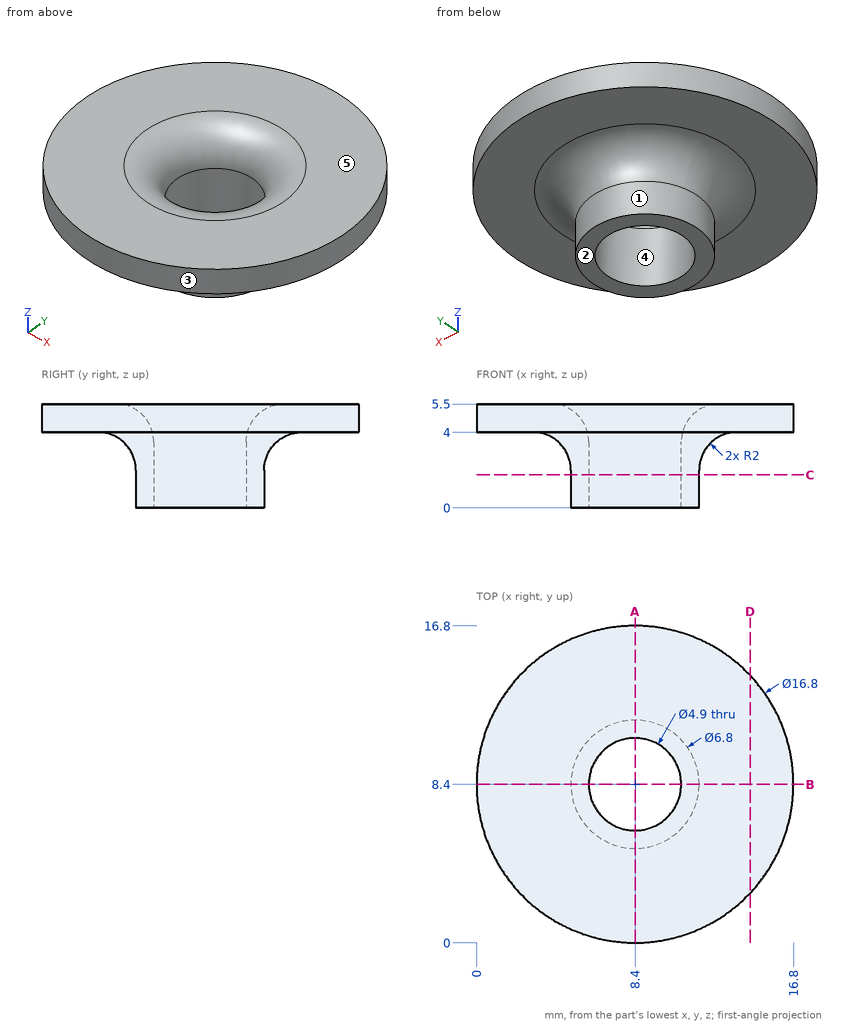
Geometry: see drawing. Coordinates: mm, zero at the bounding-box minimum. A direction names the side the tool comes from. Round coordinates to 2 decimals unless told otherwise and drop trailing zeros. Loops run counter-clockwise (first coordinate to the right, second up) from the corner with the lowest first, then second, coordinate; pieces in that order, holes last. Notation, with made-up numbers: M 28,39 L 83,39 A18 cw 83,63 Z; hole C 13,15 d9. An arc over 180 degrees is marked long. Use a Markdown table: item, result. Add a question column.
1. Section query A-A on x = 8.4. Return the cut outline in (y, z).
2. Section query D-D on x = 14.5. Return the cut outline in (y, z).
3. Mould query, pull axis X, two halves, no side actions, for the marked faces 3, 4 and 5. Classes: pulls with the +X half, pulls with the -X half, needs draft (parallel to the pull), parting line crosses it, or undercut.
4. Reachability of the marked faces 1 and 2 from +Z, -Z, +X, -X, +Y, -Y: full face, straight path, thin tool, end or side. Return the list, or none.
5. Line query: line 1 (Y direction, x = 8.4, z = 0.9); line 2 (Z direction, x = 10.75, y = 14.25); line 3 (X direction, y = 10.25, z = 4.5). Output: solid intervals per line, ascending.
6. Contact query for a flat-ended pin moving along its axis: P1, Ø6.5, axis at x = 8.4, y = 8.4, coming from the +Z side. Output: stop coordinate, or through.
7. Section query C-C on z = 1.75. Return the cut outline in (x, y), then the cut area to 3 significant figures.
Reported:
| question | item | result |
|---|---|---|
| 1 | outline | M 0,4 L 3,4 A2 cw 5,2 L 5,0 L 5.95,0 L 5.95,3.5 A2 ccw 3.95,5.5 L 0,5.5 Z; M 10.85,0 L 11.8,0 L 11.8,2 A2 cw 13.8,4 L 16.8,4 L 16.8,5.5 L 12.85,5.5 A2 ccw 10.85,3.5 Z |
| 2 | outline | M 2.63,4 L 14.17,4 L 14.17,5.5 L 2.63,5.5 Z |
| 3 | face 3 | parting line crosses it |
| 3 | face 4 | undercut |
| 3 | face 5 | needs draft |
| 4 | face 1 | -Z |
| 4 | face 2 | -Z, +X, -X, +Y, -Y |
| 5 | line 1 | y = 5 to 5.95, 10.85 to 11.8 |
| 5 | line 2 | z = 4 to 5.5 |
| 5 | line 3 | x = 0.21 to 6.41, 10.39 to 16.59 |
| 6 | P1 | stops at z = 5.1 |
| 7 | outline | C 8.4,8.4 d6.8; hole C 8.4,8.4 d4.9 |
| 7 | area | 17.5 mm² |
